Drawing for the job (mm, zero at the part's lowest x, y, z). Coordinates: 2 decimals unless noted, no trailing zeros. Write each loop counter-clockwise with the first axis right and the second up, starting at its lowest first coordinate (ties: lowest second). Pieces come first, ordered by that corner, then holes. Notation, with made-up numbers: (7, 24) - (45, 24) arc R15 cw to (45, 45) - close; hole circle Ø10 at (55, 22.25). An arc over 180 degrees is marked (long way). Write each question's results on one line, items separated by ' | '.
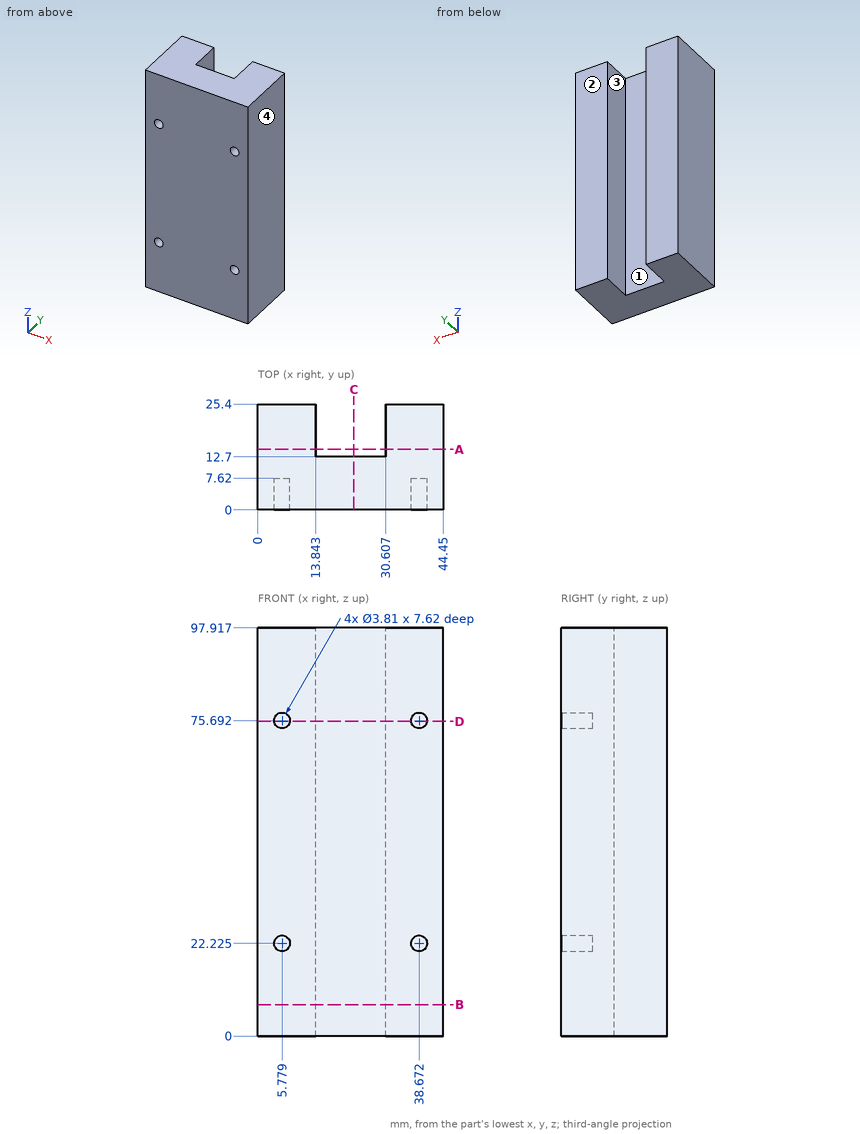
(1) Saw through at B-B on z = 7.5. Write the cut outline in (x, y), then the cut area to 3 significant figures.
Return value:
outline: (0, 0) - (44.45, 0) - (44.45, 25.4) - (30.61, 25.4) - (30.61, 12.7) - (13.84, 12.7) - (13.84, 25.4) - (0, 25.4) - close | area: 916 mm^2
(2) Saw through at C-C on x = 23. Write the cut outline in (y, z), then the cut area to 3 significant figures.
Return value:
outline: (0, 0) - (12.7, 0) - (12.7, 97.92) - (0, 97.92) - close | area: 1,240 mm^2
(3) Flat gauge pins, fed straight in: P1, Ø4, axis at x = 28, z = 34, coming from the +Y side; P2, Ø4, axis at x = 28.5, y = 4.5, coming from the -Z side; P3, Ø2.5, axis at x = 38.67, z = 75.69, coming from the -Y side. Where does each tip first touch, or does it go through?
Return value:
P1: stops at y = 12.7 | P2: stops at z = 0 | P3: stops at y = 7.62
(4) Wall check: line 1 (X direction, y = 17.5, z = 44.5); line 2 (Y direction, x = 23, z = 9). Give the ranges that are in metal, low to high. Write a range as from..to.
Return value:
line 1: x = 0..13.84, 30.61..44.45 | line 2: y = 0..12.7
(5) Saw through at A-A on y = 14.5. Write the cut outline in (x, z).
Return value:
outline: (0, 0) - (13.84, 0) - (13.84, 97.92) - (0, 97.92) - close; (30.61, 0) - (44.45, 0) - (44.45, 97.92) - (30.61, 97.92) - close
(6) Two-plate mould, pull along X, no slides. Class the marked faces 1, 2, 3 and 4: released by +X, released by -X, zero draft, split by the parting line, or undercut.
Return value:
face 1: undercut | face 2: zero draft | face 3: undercut | face 4: released by +X
(7) Saw through at D-D on z = 75.5. Write the cut outline in (x, y).
Return value:
outline: (0, 0) - (3.88, 0) - (3.88, 7.62) - (7.67, 7.62) - (7.67, 0) - (36.78, 0) - (36.78, 7.62) - (40.57, 7.62) - (40.57, 0) - (44.45, 0) - (44.45, 25.4) - (30.61, 25.4) - (30.61, 12.7) - (13.84, 12.7) - (13.84, 25.4) - (0, 25.4) - close
